Design review of the part built by this model. Coordinates are the model's own, in mm. Face numbers are marked on the shaded views. A direction names the side the tool comes from. Coordinates: 2 decimals unless noted, no trailing zeros. Loops run counter-clockwise (first coordinate to the right, second up) from the corner with the lowest first, then second, coordinate; pieces in that order, holes last. Notation, with made-up numbers: M 22,4 L 42,4 A19 ccw 42,28 Z; hole C 43,-15.5 d1. An arc over 180 degrees is marked long. Answer as a JSON object with one key per item and string values. Group by question number.
1. Machinability: for the marked faces 4, 5 and 6, which of the approach directions +Z, -Z, +X, -X, +Y, -Y give a long, thin tool a straight path to every point of the face, cutting with its end or side? Answer none if there is none.
2. Consider section D-D (x = -37). State the section outline as (y, z) points.
3. Draft analysis for pull direction X (two halves, no side actions). For the marked faces 1, 2 and 3, state which applies: +X half, -X half, draft (parallel to the pull), parting line (faces both ways), or undercut.
4. Consider section A-A (z = 15). State the section outline as (x, y) points, then the cut area to 3 significant figures.
5. Consider section B-B (y = -3). State the section outline as (x, z) points, then the cut area to 3 significant figures.
6. Insertion check: pin 1 (7.5 mm diameter, centred on y = -0.5, z = 5, fed in from +X); pin 2 (12 mm diameter, centred on x = -28, z = 44.5, fed in from +Y); pin 3 (1.9 mm diameter, centred on x = -73.01, y = 28.09, fed in from +Z); pin 4 (2.5 mm diameter, centred on x = -72, y = -36, fed in from +Z). Each pin has a flat end and moves straight along its axis. Give the tip position at first contact, or say it passes through.
7. To check wall thickness, follow probe 1 along X at (y, z) = (4.5, 48); probe 2 along Y at (x, z) = (2, 30.5); probe 3 along Z at (x, y) = (-52.5, -29.5). State the ranges of each line that lie inside material, in increasing order.
8. Consider section C-C (z = 42.5). State the section outline as (x, y) points, then the cut area to 3 significant figures.
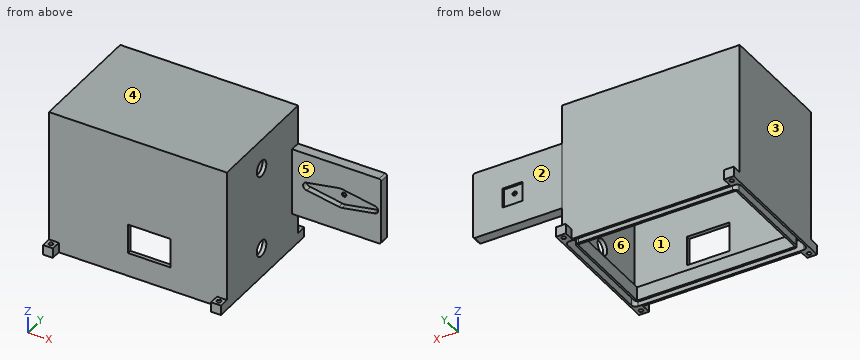
from build123d import *

# Parameters (mm, degrees)
SKETCH_1_W           = 135
SKETCH_1_H           = 60
EXTRUDE_1_DEPTH      = 70
SKETCH_6_W           = 45
SKETCH_6_H           = 70
CUT_EXTRUDE_1_DEPTH  = 0.1
SKETCH_5_W           = 45
SKETCH_5_H           = 70
CUT_EXTRUDE_2_DEPTH  = 54.9
SKETCH_7_W           = 80
SKETCH_7_H           = 50
CUT_EXTRUDE_3_DEPTH  = 75
CUT_EXTRUDE_4_DEPTH  = 6
SKETCH_10_W          = 21.5
SKETCH_10_H          = 15
CUT_EXTRUDE_6_DEPTH  = 10
SKETCH_12_W          = 18.906228009
SKETCH_12_H          = 30.34929214
CUT_EXTRUDE_7_DEPTH  = 50
CUT_EXTRUDE_8_DEPTH  = 3
SKETCH_15_W          = 10
SKETCH_15_H          = 10
CUT_EXTRUDE_9_DEPTH  = 1
SKETCH_17_R          = 1.095275866
CUT_EXTRUDE_11_DEPTH = 7
SKETCH_18_W          = 5
SKETCH_18_H          = 5
SKETCH_18_R          = 1.05
EXTRUDE_2_DEPTH      = 5
SKETCH_19_W          = 90
SKETCH_19_H          = 60
EXTRUDE_3_DEPTH      = 2
SKETCH_20_R          = 4
CUT_EXTRUDE_12_DEPTH = 10
SKETCH_21_W          = 86
SKETCH_21_H          = 56
CUT_EXTRUDE_13_DEPTH = 63
FILLET_3_R           = 1
FILLET_4_R           = 1


with BuildPart() as part:
    # 草圖1 → 填料-伸長1 (new body)
    with BuildSketch(Plane.XY):
        with Locations((-8.008902174, -4.41011236)):
            Rectangle(SKETCH_1_W, SKETCH_1_H)
    extrude(amount=EXTRUDE_1_DEPTH)

    # 草圖6 → 除料-伸長1 (cut)
    with BuildSketch(Plane(origin=(0, 25.58988764, 0), x_dir=(1, 0, 0), z_dir=(0, 1, 0))):
        with Locations((36.991097826, -35)):
            Rectangle(SKETCH_6_W, SKETCH_6_H)
    extrude(amount=-CUT_EXTRUDE_1_DEPTH, mode=Mode.SUBTRACT)

    # 草圖5 → 除料-伸長2 (cut)
    with BuildSketch(Plane.XZ.offset(34.41011236)):
        with Locations((36.991097826, 35)):
            Rectangle(SKETCH_5_W, SKETCH_5_H)
    extrude(amount=-CUT_EXTRUDE_2_DEPTH, mode=Mode.SUBTRACT)

    # 草圖7 → 除料-伸長3 (cut)
    with BuildSketch(Plane.XY):
        with Locations((-30.508902174, -4.41011236)):
            Rectangle(SKETCH_7_W, SKETCH_7_H)
    extrude(amount=CUT_EXTRUDE_3_DEPTH, mode=Mode.SUBTRACT)

    # 草圖8 → 除料-伸長4 (cut)
    with BuildSketch(Plane(origin=(0, 0, 0), x_dir=(-1, 0, 0), z_dir=(0, 0, -1))):
        with BuildLine():
            Line((-13.491097826, 22.58988764), (-13.491097826, -31.41011236))
            ThreePointArc((-13.491097826, -31.41011236), (-12.905311388, -32.824325922), (-11.491097826, -33.41011236))
            Line((-11.491097826, -33.41011236), (72.508902174, -33.41011236))
            ThreePointArc((72.508902174, -33.41011236), (73.923115736, -32.824325922), (74.508902174, -31.41011236))
            Line((74.508902174, -31.41011236), (74.508902174, 22.58988764))
            ThreePointArc((74.508902174, 22.58988764), (73.923115736, 24.004101203), (72.508902174, 24.58988764))
            Line((72.508902174, 24.58988764), (-11.491097826, 24.58988764))
            ThreePointArc((-11.491097826, 24.58988764), (-12.905311388, 24.004101203), (-13.491097826, 22.58988764))
        make_face()
        with BuildLine():
            Line((71.508902174, -28.41011236), (71.508902174, 19.58988764))
            ThreePointArc((71.508902174, 19.58988764), (70.923115736, 21.004101203), (69.508902174, 21.58988764))
            Line((69.508902174, 21.58988764), (-8.491097826, 21.58988764))
            ThreePointArc((-8.491097826, 21.58988764), (-9.905311388, 21.004101203), (-10.491097826, 19.58988764))
            Line((-10.491097826, 19.58988764), (-10.491097826, -28.41011236))
            ThreePointArc((-10.491097826, -28.41011236), (-9.905311388, -29.824325922), (-8.491097826, -30.41011236))
            Line((-8.491097826, -30.41011236), (69.508902174, -30.41011236))
            ThreePointArc((69.508902174, -30.41011236), (70.923115736, -29.824325922), (71.508902174, -28.41011236))
        make_face(mode=Mode.SUBTRACT)
    extrude(amount=-CUT_EXTRUDE_4_DEPTH, mode=Mode.SUBTRACT)

    # 草圖10 → 除料-伸長6 (cut)
    with BuildSketch(Plane(origin=(0, -34.41011236, 0), x_dir=(-1, 0, 0), z_dir=(0, -1, 0))):
        with Locations((24.758902174, -19.5)):
            Rectangle(SKETCH_10_W, SKETCH_10_H)
    extrude(amount=-CUT_EXTRUDE_6_DEPTH, mode=Mode.SUBTRACT)

    # 草圖12 → 除料-伸長7 (cut)
    with BuildSketch(Plane(origin=(14.491097826, 0, 0), x_dir=(0, 0, -1), z_dir=(1, 0, 0))):
        with Locations((-61.464370754, 15.76453371)):
            Rectangle(SKETCH_12_W, SKETCH_12_H)
        with Locations((-8.535629247, 15.76453371)):
            Rectangle(SKETCH_12_W, SKETCH_12_H)
    extrude(amount=CUT_EXTRUDE_7_DEPTH, mode=Mode.SUBTRACT)

    # 草圖14 → 除料-伸長8 (cut)
    with BuildSketch(Plane(origin=(0, 20.48988764, 0), x_dir=(-1, 0, 0), z_dir=(0, -1, 0))):
        with BuildLine():
            Line((-38.126130034, -30.080170747), (-22.017914827, -33))
            ThreePointArc((-22.017914827, -33), (-20.017914827, -35), (-22.017914827, -37))
            Line((-22.017914827, -37), (-38.126130034, -39.919829253))
            ThreePointArc((-38.126130034, -39.919829253), (-39.017914827, -40), (-39.909699621, -39.919829253))
            Line((-39.909699621, -39.919829253), (-56.017914827, -37))
            ThreePointArc((-56.017914827, -37), (-58.017914827, -35), (-56.017914827, -33))
            Line((-56.017914827, -33), (-39.909699621, -30.080170747))
            ThreePointArc((-39.909699621, -30.080170747), (-39.017914827, -30), (-38.126130034, -30.080170747))
        make_face()
    extrude(amount=-CUT_EXTRUDE_8_DEPTH, mode=Mode.SUBTRACT)

    # 草圖15 → 除料-伸長9 (cut)
    with BuildSketch(Plane(origin=(0, 25.48988764, 0), x_dir=(1, 0, 0), z_dir=(0, 1, 0))):
        with Locations((39.491097826, -33.988743251)):
            Rectangle(SKETCH_15_W, SKETCH_15_H)
    extrude(amount=-CUT_EXTRUDE_9_DEPTH, mode=Mode.SUBTRACT)

    # 草圖17 → 除料-伸長11 (cut)
    with BuildSketch(Plane(origin=(0, 20.48988764, 0), x_dir=(-1, 0, 0), z_dir=(0, -1, 0))):
        with Locations((-39.017914827, -35)):
            Circle(SKETCH_17_R)
    extrude(amount=-CUT_EXTRUDE_11_DEPTH, mode=Mode.SUBTRACT)

    # 草圖18 → 填料-伸長2 (add)
    with BuildSketch(Plane.XY):
        with Locations((11.991097826, 28.08988764)):
            Rectangle(SKETCH_18_W, SKETCH_18_H)
        with Locations((11.991097826, 28.08988764)):
            Circle(SKETCH_18_R, mode=Mode.SUBTRACT)
        with Locations((-73.008902174, 28.08988764)):
            Rectangle(SKETCH_18_W, SKETCH_18_H)
        with Locations((-73.008902174, 28.08988764)):
            Circle(SKETCH_18_R, mode=Mode.SUBTRACT)
        with Locations((-73.008902174, -36.91011236)):
            Rectangle(SKETCH_18_W, SKETCH_18_H)
        with Locations((-73.008902174, -36.91011236)):
            Circle(SKETCH_18_R, mode=Mode.SUBTRACT)
        with Locations((11.991097826, -36.91011236)):
            Rectangle(SKETCH_18_W, SKETCH_18_H)
        with Locations((11.991097826, -36.91011236)):
            Circle(SKETCH_18_R, mode=Mode.SUBTRACT)
    extrude(amount=EXTRUDE_2_DEPTH)

    # 草圖19 → 填料-伸長3 (add)
    with BuildSketch(Plane.XY.offset(70)):
        with Locations((-30.508902174, -4.41011236)):
            Rectangle(SKETCH_19_W, SKETCH_19_H)
    extrude(amount=EXTRUDE_3_DEPTH)

    # 草圖20 → 除料-伸長12 (cut)
    with BuildSketch(Plane(origin=(14.491097826, 0, 0), x_dir=(0, 0, -1), z_dir=(1, 0, 0))):
        with Locations((-15, -5.21415213)):
            Circle(SKETCH_20_R)
        with Locations((-57, -5.21415213)):
            Circle(SKETCH_20_R)
    extrude(amount=-CUT_EXTRUDE_12_DEPTH, mode=Mode.SUBTRACT)

    # 草圖21 → 除料-伸長13 (cut)
    with BuildSketch(Plane(origin=(0, 0, 7), x_dir=(-1, 0, 0), z_dir=(0, 0, -1))):
        with Locations((30.508902174, -4.41011236)):
            Rectangle(SKETCH_21_W, SKETCH_21_H)
    extrude(amount=-CUT_EXTRUDE_13_DEPTH, mode=Mode.SUBTRACT)

    # 圓角3
    fillet_3_edges = [part.edges().sort_by_distance(p)[0] for p in [
        (59.491097826, 22.98988764, 17.988743251),
    ]]
    fillet(fillet_3_edges, radius=FILLET_3_R)

    # 圓角4
    fillet_4_edges = [part.edges().sort_by_distance(p)[0] for p in [
        (59.491097826, 22.98988764, 52.011256749),
    ]]
    fillet(fillet_4_edges, radius=FILLET_4_R)


solid = part.part
Findings below:
{
 "1": {"face 4": "+Z, +X, -X, +Y, -Y", "face 5": "+Z, -Z, +X, -Y", "face 6": "none"},
 "2": {"outline": "M -34.41,0 L -33.41,0 L -33.41,6 L -30.41,6 L -30.41,0 L -29.41,0 L -29.41,7 L -32.41,7 L -32.41,70 L 23.59,70 L 23.59,7 L 20.59,7 L 20.59,0 L 21.59,0 L 21.59,6 L 24.59,6 L 24.59,0 L 25.59,0 L 25.59,72 L -34.41,72 Z"},
 "3": {"face 1": "undercut", "face 2": "draft", "face 3": "-X half"},
 "4": {"outline": "M -75.51,-34.41 L -35.51,-34.41 L -35.51,-32.41 L -73.51,-32.41 L -73.51,23.59 L 12.49,23.59 L 12.49,-1.21 L 14.49,-1.21 L 14.49,25.59 L -75.51,25.59 Z; M -14.01,-34.41 L 14.49,-34.41 L 14.49,-9.21 L 12.49,-9.21 L 12.49,-32.41 L -14.01,-32.41 Z", "area": "525 mm^2"},
 "5": {"outline": "M -75.51,0 L -74.51,0 L -74.51,6 L -71.51,6 L -71.51,0 L -70.51,0 L -70.51,7 L -73.51,7 L -73.51,70 L 12.49,70 L 12.49,60.33 L 14.49,60.33 L 14.49,72 L -75.51,72 Z; M 9.49,0 L 10.49,0 L 10.49,6 L 13.49,6 L 13.49,0 L 14.49,0 L 14.49,11.67 L 12.49,11.67 L 12.49,7 L 9.49,7 Z; M 12.49,18.33 L 14.49,18.33 L 14.49,53.67 L 12.49,53.67 Z", "area": "439 mm^2"},
 "6": {"pin 1": "stops at x = 14.49", "pin 2": "stops at y = 25.59", "pin 3": "passes through", "pin 4": "stops at z = 5"},
 "7": {"probe 1": "x = -75.51 to -73.51, 12.49 to 14.49", "probe 2": "y = -34.41 to -32.41, 23.59 to 25.59", "probe 3": "z = 0 to 7, 70 to 72"},
 "8": {"outline": "M -75.51,-34.41 L 14.49,-34.41 L 14.49,20.49 L 59.49,20.49 L 59.49,25.49 L 14.49,25.49 L 14.49,25.59 L -75.51,25.59 Z; hole M -73.51,-32.41 L 12.49,-32.41 L 12.49,23.59 L -73.51,23.59 Z", "area": "809 mm^2"}
}
